```python
from build123d import *

# Parameters (mm, degrees)
SKETCH4_R           = 59
BOSS_EXTRUDE3_DEPTH = 2
SKETCH5_R           = 1.375
BOSS_EXTRUDE5_DEPTH = 7
SKETCH8_R           = 2.375
BOSS_EXTRUDE6_DEPTH = 2
BOSS_EXTRUDE7_DEPTH = 18
SKETCH10_R          = 7.5
CUT_EXTRUDE1_DEPTH  = 18
SKETCH12_R          = 57.5
CUT_EXTRUDE2_DEPTH  = 5
CUT_EXTRUDE3_DEPTH  = 5.5
SKETCH15_R          = 89.714021058
SKETCH15_R_2        = 57
CUT_EXTRUDE4_DEPTH  = 22
SKETCH16_R          = 62.462022857
CUT_EXTRUDE8_DEPTH  = 52
CUT_EXTRUDE9_DEPTH  = 52
SKETCH18_R          = 80.62246508
SKETCH18_R_2        = 55
CUT_EXTRUDE10_DEPTH = 10
SKETCH19_R          = 55
BOSS_EXTRUDE8_DEPTH = 2
SKETCH20_R          = 6.25
CUT_EXTRUDE11_DEPTH = 2
SKETCH21_W          = 10
SKETCH21_H          = 50
CUT_EXTRUDE12_DEPTH = 3


with BuildPart() as part:
    # Sketch4 → Boss-Extrude3 (new body)
    with BuildSketch(Plane.XY):
        Circle(SKETCH4_R)
    extrude(amount=BOSS_EXTRUDE3_DEPTH)

    # Sketch5 → Boss-Extrude5 (add)
    with BuildSketch(Plane.XY.offset(2)):
        with Locations((-22.5, 27.5)):
            Circle(SKETCH5_R)
        with Locations((22.5, 27.5)):
            Circle(SKETCH5_R)
        with Locations((22.5, -27.5)):
            Circle(SKETCH5_R)
        with Locations((-22.5, -27.5)):
            Circle(SKETCH5_R)
    extrude(amount=BOSS_EXTRUDE5_DEPTH)

    # Sketch8 → Boss-Extrude6 (add)
    with BuildSketch(Plane.XY.offset(2)):
        with Locations((-22.5, 27.5)):
            Circle(SKETCH8_R)
        with Locations((22.5, 27.5)):
            Circle(SKETCH8_R)
        with Locations((-22.5, -27.5)):
            Circle(SKETCH8_R)
        with Locations((22.5, -27.5)):
            Circle(SKETCH8_R)
    extrude(amount=BOSS_EXTRUDE6_DEPTH)

    # Sketch9 → Boss-Extrude7 (add)
    with BuildSketch(Plane.XY.offset(2)):
        with BuildLine():
            ThreePointArc((-4.745762712, 55.798546005), (0, 56), (4.745762712, 55.798546005))
            Line((4.745762712, 55.798546005), (5, 58.787753827))
            ThreePointArc((5, 58.787753827), (0, 59), (-5, 58.787753827))
            Line((-5, 58.787753827), (-4.745762712, 55.798546005))
        make_face()
        with BuildLine():
            Line((-55.798546005, 4.745762712), (-58.787753827, 5))
            ThreePointArc((-58.787753827, 5), (-59, 0), (-58.787753827, -5))
            Line((-58.787753827, -5), (-55.798546005, -4.745762712))
            ThreePointArc((-55.798546005, -4.745762712), (-56, 0), (-55.798546005, 4.745762712))
        make_face()
        with BuildLine():
            ThreePointArc((58.787753827, -5), (59, 0), (58.787753827, 5))
            Line((58.787753827, 5), (55.798546005, 4.745762712))
            ThreePointArc((55.798546005, 4.745762712), (56, 0), (55.798546005, -4.745762712))
            Line((55.798546005, -4.745762712), (58.787753827, -5))
        make_face()
        with BuildLine():
            ThreePointArc((-4.745762712, -55.798546005), (0, -56), (4.745762712, -55.798546005))
            Line((4.745762712, -55.798546005), (5, -58.787753827))
            ThreePointArc((5, -58.787753827), (0, -59), (-5, -58.787753827))
            Line((-5, -58.787753827), (-4.745762712, -55.798546005))
        make_face()
    extrude(amount=BOSS_EXTRUDE7_DEPTH)

    # Sketch10 → Cut-Extrude1 (cut)
    with BuildSketch(Plane.XY.offset(2)):
        with Locations((-40, 0)):
            Circle(SKETCH10_R)
    extrude(amount=-CUT_EXTRUDE1_DEPTH, mode=Mode.SUBTRACT)

    # Sketch12 → Cut-Extrude2 (cut)
    with BuildSketch(Plane.XY.offset(20)):
        Circle(SKETCH12_R)
    extrude(amount=-CUT_EXTRUDE2_DEPTH, mode=Mode.SUBTRACT)

    # Sketch13 → Cut-Extrude3 (cut)
    with BuildSketch(Plane(origin=(0, 0, 0), x_dir=(-1, 0, 0), z_dir=(0, 0, -1))):
        with BuildLine():
            Line((-57.243329786, 4.868644068), (-58.787753827, 5))
            ThreePointArc((-58.787753827, 5), (-59, 0), (-58.787753827, -5))
            Line((-58.787753827, -5), (-57.243329786, -4.868644068))
            ThreePointArc((-57.243329786, -4.868644068), (-57.45, 0), (-57.243329786, 4.868644068))
        make_face()
        with BuildLine():
            ThreePointArc((5, 58.787753827), (0, 59), (-5, 58.787753827))
            Line((-5, 58.787753827), (-4.868644068, 57.243329786))
            ThreePointArc((-4.868644068, 57.243329786), (0, 57.45), (4.868644068, 57.243329786))
            Line((4.868644068, 57.243329786), (5, 58.787753827))
        make_face()
        with BuildLine():
            Line((-4.868644068, -57.243329786), (-5, -58.787753827))
            ThreePointArc((-5, -58.787753827), (0, -59), (5, -58.787753827))
            Line((5, -58.787753827), (4.868644068, -57.243329786))
            ThreePointArc((4.868644068, -57.243329786), (0, -57.45), (-4.868644068, -57.243329786))
        make_face()
        with BuildLine():
            ThreePointArc((58.787753827, -5), (59, 0), (58.787753827, 5))
            Line((58.787753827, 5), (57.243329786, 4.868644068))
            ThreePointArc((57.243329786, 4.868644068), (57.45, 0), (57.243329786, -4.868644068))
            Line((57.243329786, -4.868644068), (58.787753827, -5))
        make_face()
    extrude(amount=-CUT_EXTRUDE3_DEPTH, mode=Mode.SUBTRACT)

    # Sketch15 → Cut-Extrude4 (cut)
    with BuildSketch(Plane(origin=(0, 0, 0), x_dir=(-1, 0, 0), z_dir=(0, 0, -1))):
        Circle(SKETCH15_R)
        Circle(SKETCH15_R_2, mode=Mode.SUBTRACT)
    extrude(amount=-CUT_EXTRUDE4_DEPTH, mode=Mode.SUBTRACT)

    # Sketch16 → Cut-Extrude8 (cut)
    with BuildSketch(Plane.XY.offset(2)):
        Circle(SKETCH16_R)
        with BuildLine():
            Line((55.798546005, 4.745762712), (56.794948612, 4.830508475))
            ThreePointArc((56.794948612, 4.830508475), (40.305086528, 40.305086528), (4.830508475, 56.794948612))
            Line((4.830508475, 56.794948612), (4.745762712, 55.798546005))
            ThreePointArc((4.745762712, 55.798546005), (0, 56), (-4.745762712, 55.798546005))
            Line((-4.745762712, 55.798546005), (-4.830508475, 56.794948612))
            ThreePointArc((-4.830508475, 56.794948612), (-40.305086528, 40.305086528), (-56.794948612, 4.830508475))
            Line((-56.794948612, 4.830508475), (-55.798546005, 4.745762712))
            ThreePointArc((-55.798546005, 4.745762712), (-56, 0), (-55.798546005, -4.745762712))
            Line((-55.798546005, -4.745762712), (-56.794948612, -4.830508475))
            ThreePointArc((-56.794948612, -4.830508475), (-40.305086528, -40.305086528), (-4.830508475, -56.794948612))
            Line((-4.830508475, -56.794948612), (-4.745762712, -55.798546005))
            ThreePointArc((-4.745762712, -55.798546005), (0, -56), (4.745762712, -55.798546005))
            Line((4.745762712, -55.798546005), (4.830508475, -56.794948612))
            ThreePointArc((4.830508475, -56.794948612), (40.305086528, -40.305086528), (56.794948612, -4.830508475))
            Line((56.794948612, -4.830508475), (55.798546005, -4.745762712))
            ThreePointArc((55.798546005, -4.745762712), (56, 0), (55.798546005, 4.745762712))
        make_face(mode=Mode.SUBTRACT)
    extrude(amount=CUT_EXTRUDE8_DEPTH, mode=Mode.SUBTRACT)

    # Sketch17 → Cut-Extrude9 (cut)
    with BuildSketch(Plane.XY.offset(2)):
        with BuildLine():
            Line((-5, 57), (5, 57))
            Line((5, 57), (4.806106124, 54.789609817))
            ThreePointArc((4.806106124, 54.789609817), (0, 55), (-4.806106124, 54.789609817))
            Line((-4.806106124, 54.789609817), (-5, 57))
        make_face()
        with BuildLine():
            Line((54.789609817, 4.806106124), (57, 5))
            Line((57, 5), (57, -5))
            Line((57, -5), (54.789609817, -4.806106124))
            ThreePointArc((54.789609817, -4.806106124), (55, 0), (54.789609817, 4.806106124))
        make_face()
        with BuildLine():
            Line((4.806106124, -54.789609817), (5, -57))
            Line((5, -57), (-5, -57))
            Line((-5, -57), (-4.806106124, -54.789609817))
            ThreePointArc((-4.806106124, -54.789609817), (0, -55), (4.806106124, -54.789609817))
        make_face()
        with BuildLine():
            Line((-54.789609817, -4.806106124), (-57, -5))
            Line((-57, -5), (-57, 5))
            Line((-57, 5), (-54.789609817, 4.806106124))
            ThreePointArc((-54.789609817, 4.806106124), (-55, 0), (-54.789609817, -4.806106124))
        make_face()
    extrude(amount=-CUT_EXTRUDE9_DEPTH, mode=Mode.SUBTRACT)

    # Sketch18 → Cut-Extrude10 (cut)
    with BuildSketch(Plane.XY.offset(2)):
        Circle(SKETCH18_R)
        Circle(SKETCH18_R_2, mode=Mode.SUBTRACT)
    extrude(amount=-CUT_EXTRUDE10_DEPTH, mode=Mode.SUBTRACT)

    # Sketch19 → Boss-Extrude8 (add)
    with BuildSketch(Plane.XY.offset(2)):
        Circle(SKETCH19_R)
    extrude(amount=-BOSS_EXTRUDE8_DEPTH)

    # Sketch20 → Cut-Extrude11 (cut)
    with BuildSketch(Plane.XY.offset(2)):
        with Locations((0, 44.5)):
            Circle(SKETCH20_R)
        with Locations((44.5, 0)):
            Circle(SKETCH20_R)
        with Locations((0, -44.5)):
            Circle(SKETCH20_R)
        with Locations((-44.5, 0)):
            Circle(SKETCH20_R)
    extrude(amount=-CUT_EXTRUDE11_DEPTH, mode=Mode.SUBTRACT)

    # Sketch21 → Cut-Extrude12 (cut)
    with BuildSketch(Plane.XY.offset(2)):
        with Locations((30, 0)):
            Rectangle(SKETCH21_W, SKETCH21_H)
        with Locations((-30, 0)):
            Rectangle(SKETCH21_W, SKETCH21_H)
    extrude(amount=-CUT_EXTRUDE12_DEPTH, mode=Mode.SUBTRACT)


solid = part.part
```
The listing builds one solid part. Answer for the finished solid, in the listing's coordinates (mm). A direction names the side the tool comes from. Give positions to 0.01 mm unless a question says otherwise; leave off trailing zeros. Order: outer loops, then holes, each group sorted by start corner. A loop starts at its lowest first (then second) coordinate and runs counter-clockwise, first axis right, second up. Notation, with made-up numbers: (87, -4.75) - (125, -4.75) arc R38 cw to (125, 34.25) - close; hole circle Ø7 at (-27, 88). An arc over 180 degrees is marked (long way). Use one line per item in the form item = value. Start each with the question number.
(1) A cutting plane is placed at B-B, the plane y = 0. Write down the section's boundary in (x, z), then the cut area to 3 significant figures.
(2) A cutting plane is placed at A-A, the plane x = 0. Write down the section's boundary in (y, z).
(3) A cutting plane is placed at C-C, the plane y = -20.5. Write down the section's boundary in (x, z), then the cut area to 3 significant figures.
(4) Flat-ended cylindrical pins translate along their axes: pin 1 Ø11 at (x, y) = (0, 44.5) entering from -Z; pin 2 Ø1.6 at (x, z) = (-30.5, 1.5) entering from -Y; pin 3 Ø14.5 at (x, y) = (44.5, 0) entering from -Z; pin 4 Ø14.5 at (x, y) = (-44.5, 0) entering from +Z. Find the tip coordinate at first contact, or state that the pin passes through.
(5) A cutting plane is placed at D-D, the plane x = 44.5. Write down the section's boundary in (y, z), then the cut area to 3 significant figures.
(6) The mould has two halves that part along Y. Classify faces 3 (the cylindrical face through (21.487, -26.571, 6.465)), 4 (the flat face through (-1, 1, 0)): released by +Y, released by -Y, zero draft, split by the parting line, or undercut.
(7) For faces 1 (the cylindrical face through (-0.8, -38.3, 1)), 2 (the cylindrical face through (-23.513, 28.429, 6.465)), determine the directions among +Z, -Z, +X, -X, +Y, -Y from which every point of the face is accessible in a straight line to the end or side of a thin tool.
(8) Consider line 1 (Y direction, x = 0, z = 1.3); line 2 (Z direction, x = -39.5, y = 16); line 3 (X direction, y = 15, z = 1.25). Determine where each line is inside the solid, lowest interval first. Write a range as from..to.
Ans:
q1.outline = (-55, 0) - (-50.75, 0) - (-50.75, 2) - (-55, 2) - close; (-38.25, 0) - (-35, 0) - (-35, 2) - (-38.25, 2) - close; (-25, 0) - (25, 0) - (25, 2) - (-25, 2) - close; (35, 0) - (38.25, 0) - (38.25, 2) - (35, 2) - close; (50.75, 0) - (55, 0) - (55, 2) - (50.75, 2) - close
q1.area = 130 mm^2
q2.outline = (-55, 0) - (-50.75, 0) - (-50.75, 2) - (-55, 2) - close; (-38.25, 0) - (38.25, 0) - (38.25, 2) - (-38.25, 2) - close; (50.75, 0) - (55, 0) - (55, 2) - (50.75, 2) - close
q3.outline = (-51.04, 0) - (-35, 0) - (-35, 2) - (-51.04, 2) - close; (-25, 0) - (25, 0) - (25, 2) - (-25, 2) - close; (35, 0) - (51.04, 0) - (51.04, 2) - (35, 2) - close
q3.area = 164 mm^2
q4.pin_1 = through
q4.pin_2 = -46.29
q4.pin_3 = 0
q4.pin_4 = 2
q5.outline = (-32.32, 0) - (-6.25, 0) - (-6.25, 2) - (-32.32, 2) - close; (6.25, 0) - (32.32, 0) - (32.32, 2) - (6.25, 2) - close
q5.area = 104 mm^2
q6.face_3 = undercut
q6.face_4 = zero draft
q7.face_1 = +Z, -Z
q7.face_2 = +Z
q8.line_1 = -55..-50.75, -38.25..38.25, 50.75..55
q8.line_2 = 0..2
q8.line_3 = -52.92..-35, -25..25, 35..52.92
